from build123d import *

# Parameters (mm, degrees)
SKETCH_1_W          = 1590
SKETCH_1_H          = 585
EXTRUDE_1_DEPTH     = 2
EXTRUDE_2_DEPTH     = 140
SKETCH_3_W          = 1590
SKETCH_3_H          = 2
EXTRUDE_3_DEPTH     = 20
EXTRUDE_4_DEPTH     = 20
EXTRUDE_5_DEPTH     = 140
CUT_EXTRUDE_1_DEPTH = 138
SKETCH_8_W          = 20
SKETCH_8_H          = 3
EXTRUDE_6_DEPTH     = 581
SKETCH_9_W          = 3
SKETCH_9_H          = 80
EXTRUDE_7_DEPTH     = 581


with BuildPart() as part:
    # 草图1 → 凸台-拉伸1 (new body)
    with BuildSketch(Plane.XY):
        Rectangle(SKETCH_1_W, SKETCH_1_H)
    extrude(amount=EXTRUDE_1_DEPTH)

    # 草图2 → 凸台-拉伸2 (add)
    with BuildSketch(Plane.XY.offset(2)):
        Polygon((-795, -290.5), (793, -290.5), (793, 290.5), (-795, 290.5), (-795, 292.5), (795, 292.5), (795, -292.5), (-795, -292.5), align=None)
    extrude(amount=EXTRUDE_2_DEPTH)

    # 草图3 → 凸台-拉伸3 (add)
    with BuildSketch(Plane.XZ.offset(292.5)):
        with Locations((0, 141)):
            Rectangle(SKETCH_3_W, SKETCH_3_H)
    extrude_3 = extrude(amount=EXTRUDE_3_DEPTH)

    # 镜向1: 凸台-拉伸3 across plane
    add(extrude_3.mirror(Plane.ZX))

    # 草图4 → 凸台-拉伸4 (add)
    with BuildSketch(Plane(origin=(795, 0, 0), x_dir=(0, 0, -1), z_dir=(1, 0, 0))):
        Polygon((-140, 292.5), (-140, -292.5), (-140, -312.5), (-142, -312.5), (-142, 312.5), (-140, 312.5), align=None)
    extrude(amount=EXTRUDE_4_DEPTH)

    # 草图5 → 凸台-拉伸5 (add)
    with BuildSketch(Plane(origin=(0, 0, 0), x_dir=(-1, 0, 0), z_dir=(0, 0, -1))):
        with BuildLine():
            Line((795, 292.5), (795, -292.5))
            ThreePointArc((795, -292.5), (881.764191445, -375.573491887), (934.56290386, -483.469395139))
            ThreePointArc((934.56290386, -483.469395139), (981.860032363, -526.426096766), (1035.791420617, -492.166763143))
            ThreePointArc((1035.791420617, -492.166763143), (1047.805683522, -59.200609736), (795, 292.5))
        make_face()
    extrude(amount=-EXTRUDE_5_DEPTH)

    # 草图6 → 切除-拉伸1 (cut)
    with BuildSketch(Plane.XY.offset(140)):
        with BuildLine():
            Line((-797, -291.43118398), (-795, -290.5))
            Line((-795, -290.5), (-795, 290.5))
            Line((-795, 290.5), (-797, 288.591040402))
            ThreePointArc((-797, 288.591040402), (-1046.463523913, -61.653894645), (-1033.91490125, -491.474899668))
            ThreePointArc((-1033.91490125, -491.474899668), (-981.983290729, -524.429295604), (-936.512623715, -483.013081096))
            ThreePointArc((-936.512623715, -483.013081096), (-883.723814588, -374.866159142), (-797, -291.43118398))
        make_face()
    extrude(amount=-CUT_EXTRUDE_1_DEPTH, mode=Mode.SUBTRACT)

    # 草图8 → 凸台-拉伸6 (add)
    with BuildSketch(Plane.XZ.offset(-290.5)):
        with Locations((-180.065727279, 108.071414122)):
            Rectangle(SKETCH_8_W, SKETCH_8_H)
        with Locations((230.676945024, 108.071414122)):
            Rectangle(SKETCH_8_W, SKETCH_8_H)
    extrude(amount=EXTRUDE_6_DEPTH)

    # 草图9 → 凸台-拉伸7 (add)
    with BuildSketch(Plane.XZ.offset(-290.5)):
        with Locations((514.5, 102)):
            Rectangle(SKETCH_9_W, SKETCH_9_H)
    extrude(amount=EXTRUDE_7_DEPTH)


solid = part.part
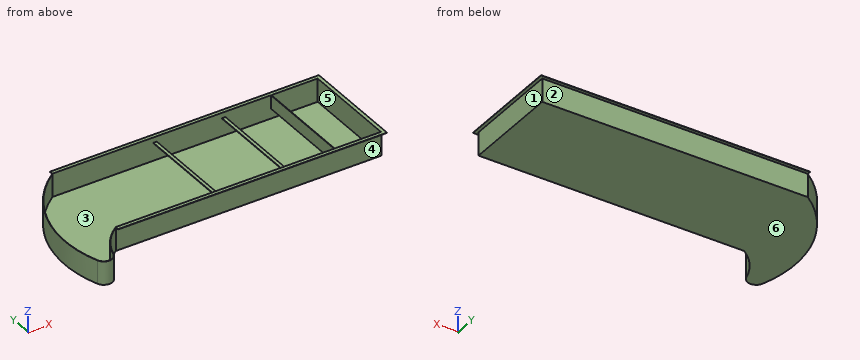
Here's how the part is built. I have some questions about the finished solid (model axes, mm). Face numbers are marked on the shaded views. A direction names the side the tool comes from. Round coordinates to 2 decimals unless told otherwise and drop trailing zeros. Write each loop counter-clockwise with the first axis right and the second up, starting at its lowest first coordinate (ties: lowest second). Pieces come first, ordered by that corner, then holes.
1. Suppose I cut it at B-B (y = 91). List the corners of the cut face in (x, z) for me.
2. Suppose I cut it at D-D (y = -206). List the corners of the cut face in (x, z) for me.
3. For the marked faces 5 and 6, which set-ups out of +Z, -Z, +X, -X, +Y, -Y let a thin tool reach every point of the face, with its end or its side?
4. Suppose I cut it at A-A (z = 37.5). List the corners of the cut face in (x, y) for me (3 decimals), and give its area (3 significant figures).
5. I need wall thicknesses on L1, parallel to Y at x = 292.5, z = 115; L2, parallel to X at y = 247.5, z = 72.5; L3, parallel to X at y = -224, z = 89.5. Which ranges of each line are inside material? Lowest first, please.
6. Suppose I cut it at C-C (x = 475.5). List the corners of the cut face in (y, z) for me, and give its area (3 significant figures).
7. Will these pins go through, and if not, where does the flat tip stop? pin 1 Ø6 at (x, z) = (-193.5, 33.5) entering from -Y; pin 2 Ø0.6 at (y, z) = (300.5, 140.5) entering from -X; pin 3 Ø6 at (x, y) = (-182, 112.5) entering from -Z; pin 4 Ø1.6 at (x, z) = (5, 141) entering from -Y.
8. If we mould it in two halves opening along Y, with no side actions, what happens to the marked faces 1, 2, 3 and 4? For each: released by +Y, released by -Y, zero draft, split by the parting line, or undercut.
Answer sheet:
1. outline: (-980.83, 0) - (795, 0) - (795, 140) - (815, 140) - (815, 142) - (793, 142) - (793, 2) - (-978.49, 2) - (-978.49, 140) - (-980.83, 140) - close; (-190.07, 106.57) - (-170.07, 106.57) - (-170.07, 109.57) - (-190.07, 109.57) - close; (220.68, 106.57) - (240.68, 106.57) - (240.68, 109.57) - (220.68, 109.57) - close; (513, 62) - (516, 62) - (516, 142) - (513, 142) - close
2. outline: (-1075.61, 0) - (795, 0) - (795, 140) - (815, 140) - (815, 142) - (793, 142) - (793, 2) - (-1073.61, 2) - (-1073.61, 140) - (-1075.61, 140) - close; (-190.07, 106.57) - (-170.07, 106.57) - (-170.07, 109.57) - (-190.07, 109.57) - close; (220.68, 106.57) - (240.68, 106.57) - (240.68, 109.57) - (220.68, 109.57) - close; (513, 62) - (516, 62) - (516, 142) - (513, 142) - close
3. face 5: +Z
3. face 6: -Z, +X, -X, +Y, -Y
4. outline: (-1035.791, -492.167) arc R52.674 ccw to (-934.563, -483.469) arc R342.989 cw to (-795, -292.5) - (795, -292.5) - (795, 292.5) - (-795, 292.5) arc R677.25 ccw to start; hole (-1033.915, -491.475) arc R50.674 ccw to (-936.513, -483.013) arc R344.989 cw to (-797, -291.431) - (-795, -290.5) - (793, -290.5) - (793, 290.5) - (-795, 290.5) - (-797, 288.591) arc R675.25 ccw to start
4. area: 10,000 mm2
5. L1: y = -292.5 to -290.5, 290.5 to 292.5
5. L2: x = -851.19 to -848.18, 513 to 516, 793 to 795
5. L3: x = -1076.76 to -1074.75, 513 to 516, 793 to 795
6. outline: (-312.5, 140) - (-292.5, 140) - (-292.5, 0) - (292.5, 0) - (292.5, 140) - (312.5, 140) - (312.5, 142) - (290.5, 142) - (290.5, 2) - (-290.5, 2) - (-290.5, 142) - (-312.5, 142) - close
6. area: 1,810 mm2
7. pin 1: stops at y = -292.5
7. pin 2: stops at x = -795
7. pin 3: stops at z = 0
7. pin 4: stops at y = -312.5
8. face 1: zero draft
8. face 2: released by +Y
8. face 3: undercut
8. face 4: released by -Y
